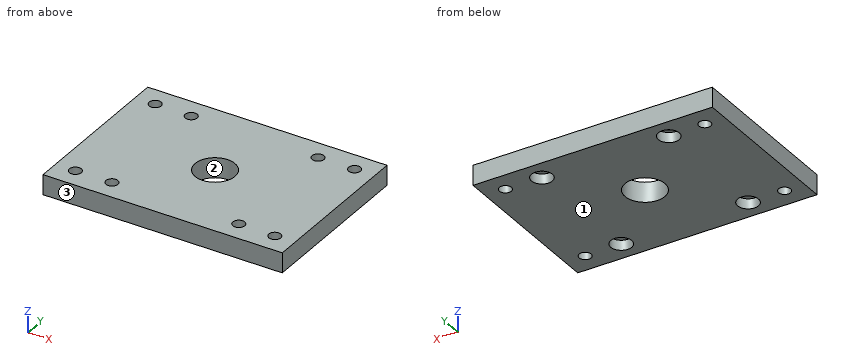
```python
from build123d import *

# Parameters (mm, degrees)
SKETCH1_W           = 60
SKETCH1_H           = 42
SKETCH1_R           = 1.5
SKETCH1_R_2         = 5
BOSS_EXTRUDE1_DEPTH = 5
SKETCH3_R           = 2.625
CUT_EXTRUDE4_DEPTH  = 2.5


with BuildPart() as part:
    # Sketch1 → Boss-Extrude1 (new body)
    with BuildSketch(Plane.XY):
        Rectangle(SKETCH1_W, SKETCH1_H)
        with Locations((-15.9, 15.9)):
            Circle(SKETCH1_R, mode=Mode.SUBTRACT)
        with Locations((15.9, 15.9)):
            Circle(SKETCH1_R, mode=Mode.SUBTRACT)
        with Locations((15.9, -15.9)):
            Circle(SKETCH1_R, mode=Mode.SUBTRACT)
        with Locations((-15.9, -15.9)):
            Circle(SKETCH1_R, mode=Mode.SUBTRACT)
        with Locations((-25, 16)):
            Circle(SKETCH1_R, mode=Mode.SUBTRACT)
        Circle(SKETCH1_R_2, mode=Mode.SUBTRACT)
        with Locations((25, 16)):
            Circle(SKETCH1_R, mode=Mode.SUBTRACT)
        with Locations((25, -16)):
            Circle(SKETCH1_R, mode=Mode.SUBTRACT)
        with Locations((-25, -16)):
            Circle(SKETCH1_R, mode=Mode.SUBTRACT)
    extrude(amount=BOSS_EXTRUDE1_DEPTH)

    # Sketch3 → Cut-Extrude4 (cut)
    with BuildSketch(Plane(origin=(0, 0, 0), x_dir=(-1, 0, 0), z_dir=(0, 0, -1))):
        with Locations((-15.9, 15.9)):
            Circle(SKETCH3_R)
        with Locations((15.9, 15.9)):
            Circle(SKETCH3_R)
        with Locations((15.9, -15.9)):
            Circle(SKETCH3_R)
        with Locations((-15.9, -15.9)):
            Circle(SKETCH3_R)
    extrude(amount=-CUT_EXTRUDE4_DEPTH, mode=Mode.SUBTRACT)


solid = part.part
```
The model under review builds one solid part; all positions refer to its coordinate system, in mm. Face numbers are marked on the shaded views. Round coordinates to 2 decimals unless told otherwise and drop trailing zeros. Loops run counter-clockwise (first coordinate to the right, second up) from the corner with the lowest first, then second, coordinate; pieces in that order, holes last.
1) The part is to be moulded in two halves that separate along Y. For the marked faces 1, 2 and 3, say which applies: pulls with the +Y half, pulls with the -Y half, needs draft (parallel to the pull), parting line crosses it, or undercut.
Values follow:
face 1: needs draft
face 2: undercut
face 3: pulls with the -Y half
2) Clearance check with flat-ended pins moving along their axes: P1, Ø9, axis at x = 0, y = 0, coming from the -Z side; P2, Ø1.6, axis at x = 15, y = 17, coming from the -Z side. State where each tip first meets the part, or that it passes through.
Values follow:
P1: passes through
P2: stops at z = 2.5
3) Consider section D-D on x = -2.5. State the section outline as (y, z) points, then the cut area to 3 significant figures.
Values follow:
outline: (-21, 0) - (-4.33, 0) - (-4.33, 5) - (-21, 5) - close; (4.33, 0) - (21, 0) - (21, 5) - (4.33, 5) - close
area: 167 mm2
4) Consider section A-A on y = -3. State the section outline as (x, z) points.
Values follow:
outline: (-30, 0) - (-4, 0) - (-4, 5) - (-30, 5) - close; (4, 0) - (30, 0) - (30, 5) - (4, 5) - close
5) Consider section B-B on x = 25. State the section outline as (y, z) points, then the cut area to 3 significant figures.
Values follow:
outline: (-21, 0) - (-17.5, 0) - (-17.5, 5) - (-21, 5) - close; (-14.5, 0) - (14.5, 0) - (14.5, 5) - (-14.5, 5) - close; (17.5, 0) - (21, 0) - (21, 5) - (17.5, 5) - close
area: 180 mm2
6) Consider section C-C on z = 1. Give the number of separate pieces and of enclosed holes in the cut face, then the cut area to 3 significant figures.
Values follow:
separate pieces: 1
enclosed holes: 9
area: 2,330 mm2
7) Wall thickness on line 1 along Y through (x, z) = (-25, 2.6); line 2 along Y through (x, z) = (16, 3.75); line 3 along X through (y, z) = (15.9, 4.15): over which ranges is each line inside the solid? List them lowest first.
Values follow:
line 1: y = -21 to -17.5, -14.5 to 14.5, 17.5 to 21
line 2: y = -21 to -17.4, -14.4 to 14.4, 17.4 to 21
line 3: x = -30 to -26.5, -23.5 to -17.4, -14.4 to 14.4, 17.4 to 23.5, 26.5 to 30
